Can you work these out from the model? Positions are in its coordinate system, mm. A direction names the side the tool comes from. Round coordinates to 2 decimals unless told otherwise and drop trailing zeros. Write each loop counter-clockwise with the first axis right and the second up, starting at its lowest first coordinate (ties: lowest second). Pieces come first, ordered by that corner, then holes.
Q1. Please list where these lines run through material, in increasing order: line 1 along X through (y, z) = (1.55, 18); line 2 along Z through (x, y) = (-18, 2.2); line 3 along X through (y, z) = (2, -0.5).
Q2. I'm going to push a flat-ended pin straight in: pin 1 Ø4 at (y, z) = (-0.5, 26) entering from -X. Where does the tip first touch, or does it pass through?
Q3. For faces 5 (the flat face through (-65, 2, -15)), 6 (the flat face through (97, -8, 40)), 7 (the flat face through (97, -4, -37.5)), which set-ups out of +Z, -Z, +X, -X, +Y, -Y let a thin tool reach every point of the face, with its end or its side?
Q4. If we section it at D-D (z = 5.5): Please give me the cut outline in (x, y).
Q5. If we section it at B-B (y = -5): Give the number of separate pieces and of enclosed holes in the cut face, plus the area to 3 significant figures.
Q6. We'd pull the mould along X, two halves only. Please class faces 1 (the flat face through (99, 1, 10)), 2 (the flat face through (-97, -8, 40)), 3 (the flat face through (55, 2, -15)), 4 (the flat face through (-94, -3, -40)): +X half, -X half, draft (parallel to the pull), parting line (faces both ways), or undercut.
Q7. If we section it at C-C (x = -75): Please give me the cut outline in (y, z).
Q8. If we section it at A-A (z = -15): Please give me the cut outline in (x, y).
from build123d import *

# Parameters (mm, degrees)
SKETCH_1_W          = 198
SKETCH_1_H          = 85
EXTRUDE_1_DEPTH     = 3
SKETCH_3_W          = 4.997331483
SKETCH_3_H          = 8
SKETCH_3_R          = 1.65
SKETCH_3_W_2        = 5
EXTRUDE_2_DEPTH     = 5
SKETCH_4_W          = 5
SKETCH_4_H          = 8
SKETCH_4_R          = 1.65
EXTRUDE_3_DEPTH     = 5
SKETCH_5_R          = 1.25
CUT_EXTRUDE_1_DEPTH = 10
CUT_EXTRUDE_2_DEPTH = 3


with BuildPart() as part:
    # 草图1 → 凸台-拉伸1 (new body)
    with BuildSketch(Plane(origin=(0, 0, 0), x_dir=(1, 0, 0), z_dir=(0, 1, 0))):
        Rectangle(SKETCH_1_W, SKETCH_1_H)
    extrude(amount=EXTRUDE_1_DEPTH)

    # 草图3 → 凸台-拉伸2 (add)
    with BuildSketch(Plane.ZY.offset(99)):
        with Locations((-40.001334259, -4)):
            Rectangle(SKETCH_3_W, SKETCH_3_H)
        with Locations((-40, -5)):
            Circle(SKETCH_3_R, mode=Mode.SUBTRACT)
        with Locations((40, -4)):
            Rectangle(SKETCH_3_W_2, SKETCH_3_H)
        with Locations((40, -5)):
            Circle(SKETCH_3_R, mode=Mode.SUBTRACT)
    extrude(amount=-EXTRUDE_2_DEPTH)

    # 草图4 → 凸台-拉伸3 (add)
    with BuildSketch(Plane(origin=(99, 0, 0), x_dir=(0, 0, -1), z_dir=(1, 0, 0))):
        with Locations((-40, -4)):
            Rectangle(SKETCH_4_W, SKETCH_4_H)
        with Locations((-40, -5)):
            Circle(SKETCH_4_R, mode=Mode.SUBTRACT)
        with Locations((40, -4)):
            Rectangle(SKETCH_4_W, SKETCH_4_H)
        with Locations((40, -5)):
            Circle(SKETCH_4_R, mode=Mode.SUBTRACT)
    extrude(amount=-EXTRUDE_3_DEPTH)

    # 草图5 → 切除-拉伸1 (cut)
    with BuildSketch(Plane(origin=(0, 3, 0), x_dir=(1, 0, 0), z_dir=(0, 1, 0))):
        with Locations((-18, 18)):
            Circle(SKETCH_5_R)
        with Locations((-18, -18)):
            Circle(SKETCH_5_R)
        with Locations((18, -18)):
            Circle(SKETCH_5_R)
        with Locations((18, 18)):
            Circle(SKETCH_5_R)
    extrude(amount=-CUT_EXTRUDE_1_DEPTH, mode=Mode.SUBTRACT)

    # 草图6 → 切除-拉伸2 (cut)
    with BuildSketch(Plane(origin=(0, 3, 0), x_dir=(1, 0, 0), z_dir=(0, 1, 0))):
        Polygon((60, 30), (70, 30), (40, 0), (30, 0), align=None)
        Polygon((-40, 0), (-30, 0), (-60, 30), (-70, 30), align=None)
        Polygon((-60, 0), (-50, 0), (-80, 30), (-90, 30), align=None)
        Polygon((80, 30), (90, 30), (60, 0), (50, 0), align=None)
    extrude(amount=-CUT_EXTRUDE_2_DEPTH, mode=Mode.SUBTRACT)


solid = part.part
A:
1. line 1: x = -99 to -19.25, -16.75 to 16.75, 19.25 to 99
1. line 2: z = -42.5 to -19.25, -16.75 to 16.75, 19.25 to 42.5
1. line 3: x = -99 to -60.5, -50.5 to -40.5, -30.5 to 30.5, 40.5 to 50.5, 60.5 to 99
2. pin 1: stops at x = -99
3. face 5: +Y, -Y
3. face 6: +Z, -Z, +X, -X, -Y
3. face 7: +X, -X, -Y
4. outline: (-99, 0) - (99, 0) - (99, 3) - (-99, 3) - close
5. separate pieces: 8
5. enclosed holes: 0
5. area: 34.0 mm2
6. face 1: +X half
6. face 2: draft
6. face 3: undercut
6. face 4: undercut
7. outline: (0, -42.5) - (3, -42.5) - (3, -25) - (0, -25) - close; (0, -15) - (3, -15) - (3, 42.5) - (0, 42.5) - close
8. outline: (-99, 0) - (-75, 0) - (-75, 3) - (-99, 3) - close; (-65, 0) - (-55, 0) - (-55, 3) - (-65, 3) - close; (-45, 0) - (45, 0) - (45, 3) - (-45, 3) - close; (55, 0) - (65, 0) - (65, 3) - (55, 3) - close; (75, 0) - (99, 0) - (99, 3) - (75, 3) - close
